Autodesk Fusion 360 part; units mm, degrees
sketch "Sketch1" plane through (0, 0, 0) normal (0, 0, 1) x (1, 0, 0)
  line L0 (-5.4993, 9.525) -> (-10.9985, 0)
  line L1 (-10.9985, 0) -> (-5.4993, -9.525)
  line L2 (-5.4993, -9.525) -> (5.4993, -9.525)
  line L3 (5.4993, -9.525) -> (10.9985, 0)
  line L4 (10.9985, 0) -> (5.4993, 9.525)
  line L5 (5.4993, 9.525) -> (-5.4993, 9.525)
  line L6 (-8.386, -14.525) -> (8.386, -14.525)
  line L7 (8.386, -14.525) -> (16.772, 0)
  line L8 (16.772, 0) -> (8.386, 14.525)
  line L9 (8.386, 14.525) -> (-8.386, 14.525)
  line L10 (-8.386, 14.525) -> (-16.772, 0)
  line L11 (-16.772, 0) -> (-8.386, -14.525)
  dimension "d1" = 19.05
  dimension "d2" = 5
extrude "Extrude1" add sketch "Sketch1" along normal blind 6.35
sketch "Sketch2" plane through (0, 0, 6.35) normal (0, 0, 1) x (-1, 0, 0)
  line L0 (5.4993, -9.525) -> (-5.4993, -9.525)
  line L1 (-5.4993, -9.525) -> (-10.9985, 0)
  line L2 (-10.9985, 0) -> (-5.4993, 9.525)
  line L3 (-5.4993, 9.525) -> (5.4993, 9.525)
  line L4 (5.4993, 9.525) -> (10.9985, 0)
  line L5 (10.9985, 0) -> (5.4993, -9.525)
  line L6 (16.772, 0) -> (8.386, 14.525)
  line L7 (8.386, 14.525) -> (-8.386, 14.525)
  line L8 (-8.386, 14.525) -> (-16.772, 0)
  line L9 (-16.772, 0) -> (-8.386, -14.525)
  line L10 (-8.386, -14.525) -> (8.386, -14.525)
  line L11 (8.386, -14.525) -> (16.772, 0)
  line L12 (1.5, -9.525) -> (1.5, -2.5981)
  line L13 (1.5, -2.5981) -> (7.4989, -6.0615)
  line L14 (1.5, -6.0615) -> (4.4994, -4.3298)
  dimension "d5" = 1.5
extrude "Extrude2" add sketch "Sketch2" against normal up to surface (6.35 mm away) contours L0 L5 L12 L13 L14
pattern_circular "C-Pattern1" count 6 over 360 about axis through (0, 0, 1.75) along (0, 0, 1) of "Extrude2"
sketch "Sketch3" plane through (0, 14.525, 0) normal (0, 1, 0) x (-1, 0, 0)
  line L0 (-8.386, 0) -> (8.386, 0)
  line L1 (8.386, 0) -> (8.386, 6.35)
  line L2 (8.386, 6.35) -> (-8.386, 6.35)
  line L3 (-8.386, 6.35) -> (-8.386, 0)
  point P0 (0, 3.175)
  point P1 (8.386, 3.175)
hole "Hole1" at (0, 14.525, 3.175) direction (0, -1, 0) diameter 2.7 end through all
pattern_circular "C-Pattern2" count 3 over 360 about axis through (0, 0, 1.75) along (0, 0, 1) of "Hole1"
sketch "Sketch4" plane through (8.2489, -4.7625, 0) normal (-0.866, 0.5, 0) x (-0.5, -0.866, 0)
  circle A0 centre (0, 3.175) radius 1.35
  line L0 (-1.5, 6.35) -> (-1.5, 0)
  line L1 (-1.5, 0) -> (1.5, 0)
  line L2 (1.5, 0) -> (1.5, 6.35)
  line L3 (1.5, 6.35) -> (-1.5, 6.35)
  line L4 (-2.55, 1.7028) -> (0, 0.2305)
  line L5 (0, 0.2305) -> (2.55, 1.7028)
  line L6 (2.55, 1.7028) -> (2.55, 4.6472)
  line L7 (2.55, 4.6472) -> (0, 6.1195)
  line L8 (0, 6.1195) -> (-2.55, 4.6472)
  line L9 (-2.55, 4.6472) -> (-2.55, 1.7028)
  line L10 (-2.55, 1.7028) -> (-2.55, 0)
  line L11 (-2.55, 0) -> (2.55, 0)
  line L12 (2.55, 0) -> (2.55, 1.7028)
  point P0 (0, 3.175)
  dimension "d15" = 5.1
extrude "Extrude3" cut sketch "Sketch4" against normal blind 2.1 contours L0 L2 L4 L5 L7 L8 | L0 L4 L8 L9 | L0 L1 L2 L4 L5 L11 | L0 L4 L10 L11 | L2 L5 L6 L7 | L2 L5 L11 L12
pattern_circular "C-Pattern3" count 6 over 360 about axis through (0, 0, 1.75) along (0, 0, 1) of "Extrude3"
Work out the finished part from the listing and answer in its coordinate system (mm). A direction names the side the tool comes from. Coordinates: 2 decimals unless noted, no trailing zeros. Write each loop counter-clockwise with the first axis right and the second up, starting at its lowest first coordinate (ties: lowest second). Pieces come first, ordered by that corner, then holes.
1. Consider line 1 along X through (y, z) = (5.5, 5); line 2 along Z through (x, y) = (0, 13.6) (3 decimals); line 3 along Y through (x, z) = (11, 4). Determine where each line is inside the solid, lowest interval first.
Results list:
line 1: x = -13.6 to -10.25, -6.53 to -2.47, 2.47 to 6.53, 10.25 to 13.6
line 2: z = 0 to 1.825, 4.525 to 6.35
line 3: y = -10 to -7.58, -5.12 to -4.2, -3.41 to 3.41, 4.2 to 5.12, 7.58 to 10
2. For faces 5 (the cylindrical face through (11.05, -6.98, 4.42)), 6 (the flat face through (-1.5, 8, 3)), 7 (the flat face through (-2.55, 11, 2)), determine the directions among +Z, -Z, +X, -X, +Y, -Y from which every point of the face is accessible in a straight line to the end or side of a thin tool.
Results list:
face 5: none
face 6: +Z, -Z
face 7: -Z
3. For a pull along Y with two mould halves and no side action, classify faces 1 (the flat face through (-10.333, -5.353, 1.743)), 2 (the flat face through (2, 9.525, 3)), 3 (the flat face through (0, 14.525, 5)), 4 (the flat face through (13.45, -5.75, 3.13)) as +Y half, -Y half, draft (parallel to the pull), parting line (faces both ways), or undercut.
Results list:
face 1: undercut
face 2: undercut
face 3: +Y half
face 4: -Y half
4. Flat-ended cylindrical pins translate along their axes: pin 1 (3 mm diameter, centred on y = -7.5, z = 3, fed in from +X); pin 2 (1.7 mm diameter, centred on y = 10.5, z = 3, fed in from +X); pin 3 (1 mm diameter, centred on y = -3.5, z = 5, fed in from -X). Find the tip coordinate at first contact, or state that the pin passes through.
Results list:
pin 1: stops at x = 13.31
pin 2: stops at x = 11.2
pin 3: stops at x = -15.04
5. The part is cut by section A-A, the plane y = 10.25. Write down the section's boundary in (x, z).
Results list:
outline: (-10.85, 0) - (-2.55, 0) - (-2.55, 4.65) - (0, 6.12) - (2.55, 4.65) - (2.55, 0) - (10.85, 0) - (10.85, 6.35) - (-10.85, 6.35) - close
